Geometry check sheet. Reference: drawing and pictorial views, mm from the part's lowest x, y, z. A direction names the side the tool comes from. Give positions to 0.01 mm unless a question says otherwise; leave off trailing zeros. Order: outer loops, then holes, each group sorted by start corner. A loop starts at its lowest first (then second) coordinate and runs counter-clockwise, first axis right, second up. Notation, with made-up numbers: M -26.75,-11.5 L -2.75,-11.5 A23 cw -2.75,9.5 Z; hole C 14,10.25 d1. An arc over 180 degrees is marked long. Answer as CSV lines item,"result". Start each with the question number.
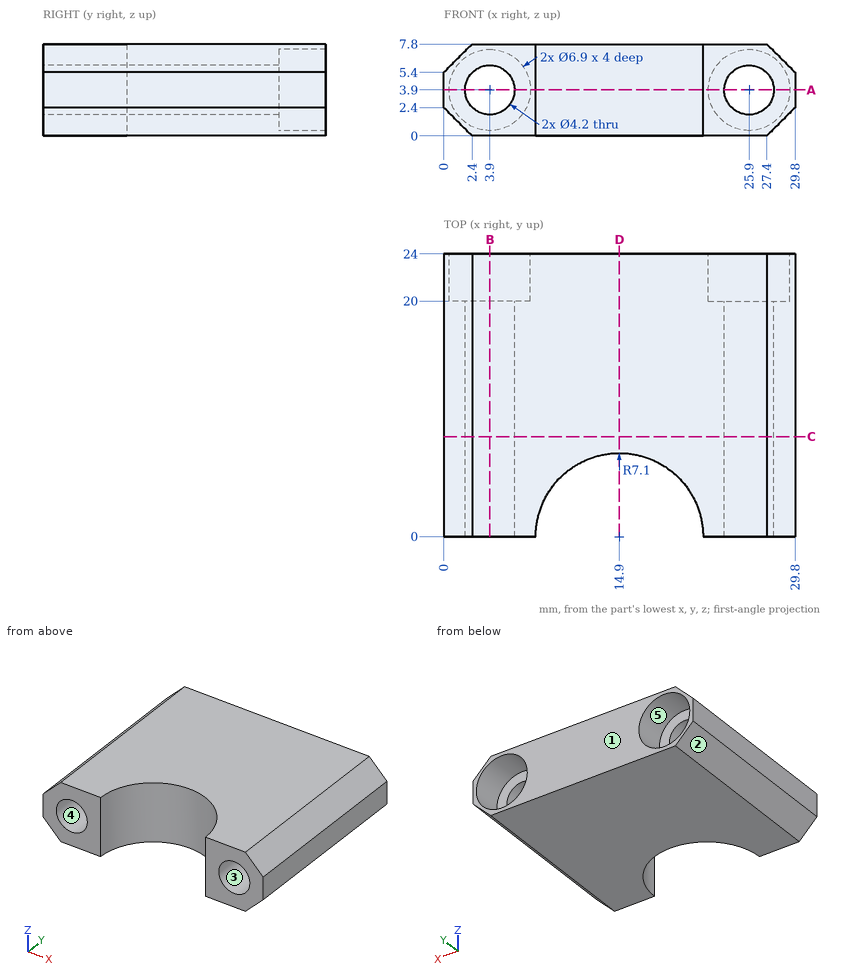
Item 1: Section check D-D on x = 14.9. Record the boundary of the cut face in (y, z), then the cut area to 3 significant figures.
Item 2: Section check C-C on y = 8.5. Record the boundary of the cut face in (x, z).
Item 3: Depth check by flat-ended pin: pin 1 Ø2 at (x, z) = (4.5, 2.5) entering from +Y; pin 2 Ø4 at (x, z) = (12.5, 4) entering from -Y. Enter the tip coordinate at first touch or a pass-through.
Item 4: Access from +Z, -Z, +X, -X, +Y, -Y to the whole of each face (thin tool, end or side, straight path). Record for the marked faces 4 and 5.
Item 5: Scan lines: line 1 along X through (y, z) = (16.25, 3.9); line 2 along X through (y, z) = (22.35, 3.9); line 3 along Z through (x, y) = (25.9, 21.8). Record each from-to range of solid material in increasing order.
Item 6: Section check A-A on z = 3.9. Record the boundary of the cut face in (x, y), then the cut area to 3 significant figures.
Item 7: Section check B-B on x = 3.9. Record the boundary of the cut face in (y, z), then the cut area to 3 significant figures.
Item 8: Draft check along X on the marked faces 1, 2 and 3. Enter one of: pulls with the +X half, pulls with the -X half, needs draft (parallel to the pull), parting line crosses it, or undercut.
Numbers:
1,outline,"M 7.1,0 L 24,0 L 24,7.8 L 7.1,7.8 Z"
1,area,"132 mm2"
2,outline,"M 0,2.4 L 2.4,0 L 27.4,0 L 29.8,2.4 L 29.8,5.4 L 27.4,7.8 L 2.4,7.8 L 0,5.4 Z; hole C 3.9,3.9 d4.2; hole C 25.9,3.9 d4.2"
3,pin 1,"y = 20"
3,pin 2,"y = 5.57"
4,face 4,"+Y, -Y"
4,face 5,"+Y"
5,line 1,"0 to 1.8, 6 to 23.8, 28 to 29.8"
5,line 2,"0 to 0.45, 7.35 to 22.45, 29.35 to 29.8"
5,line 3,"0 to 0.45, 7.35 to 7.8"
6,outline,"M 0,0 L 1.8,0 L 1.8,20 L 0.45,20 L 0.45,24 L 0,24 Z; M 6,0 L 7.8,0 A7.1 cw 22,0 L 23.8,0 L 23.8,20 L 22.45,20 L 22.45,24 L 7.35,24 L 7.35,20 L 6,20 Z; M 28,0 L 29.8,0 L 29.8,24 L 29.35,24 L 29.35,20 L 28,20 Z"
6,area,"413 mm2"
7,outline,"M 0,0 L 24,0 L 24,0.45 L 20,0.45 L 20,1.8 L 0,1.8 Z; M 0,6 L 20,6 L 20,7.35 L 24,7.35 L 24,7.8 L 0,7.8 Z"
7,area,"75.6 mm2"
8,face 1,"needs draft"
8,face 2,"pulls with the -X half"
8,face 3,"undercut"
